Input: part model. Units: mm. Frame: model coordinates. A direction names the side the tool comes from. Give positions to 0.01 mm unless a question says otherwise; leave off trailing zeros. Loops run counter-clockwise (first coordinate to the right, second up) from the corner with the lowest first, then second, coordinate; pieces in that order, holes last. Notation, with made-up numbers: (32.25, 75) - (87.25, 75) arc R18 ccw to (87.25, 107) - close; hole circle Ø4 at (-21, 79). An arc over 180 degrees is marked (long way). Answer as a JSON object with one key per item and string values. Group by question number.
(1) Section query D-D (z = 6). Return loops of the section in (x, y) (3 decimals).
(2) Access query for faces 4 (the cylindrical face through (-7.074, 7.09, 7.535)), 5 (the flat face through (-7.375, 0, 7)), 6 (the flat face through (6.375, 0, 6)), 7 (the cylindrical face through (7.09, 7.074, 7.535)). Directions: +Z, -Z, +X, -X, +Y, -Y. A direction counts if a zero-diameter tool reaches every point of the face in a straight line with its end or side. Return the directions, or none.
(3) Mould query, pull axis Y, two halves, no side actions, for faces 1 (the flat face through (0, 0, 2)), 2 (the cylindrical face through (14.1, -14.14, 2.54)), 3 (the flat face through (0, 10, 5)). Classes: +Y half, -Y half, draft (parallel to the pull), parting line (faces both ways), or undercut.
(4) Section query B-B (y = 5). Return loops of the section in (x, z) (3 decimals).
(5) Section query A-A (z = 3). Return loops of the section in (x, y) (3 decimals).
(6) Material intervals for L1, parallel to X at y = 0.75, z = 4.5 (3 decimals); L2, parallel to Y at x = 0, z = 7.25 (3 decimals), sorted ascending.
(7) Section query C-C (x = 6.75). Return loops of the section in (y, z), plus the area to 3 significant figures.
(8) Pin query (flat end, axial travel): P1, Ø4, axis at y = -0.5, z = 7.5, coming from the -X side (3 decimals); P2, Ø1.5, axis at y = -2.5, z = 7, coming from the +X side (3 decimals); P3, Ø2.5, axis at x = -2.5, z = 7.5, coming from the +Y side (3 decimals). Return the tip coordinate at first contact, or that it passes through.
Autodesk Fusion 360 part; units mm, degrees
sketch "Sketch1" plane through (0, 0, 0) normal (0, 0, 1) x (1, 0, 0)
  line L0 (15, -15) -> (-15, -15)
  line L1 (-15, -15) -> (-15, 15)
  line L2 (-15, 15) -> (15, 15)
  line L3 (15, 15) -> (15, -15)
  line L4 (15, -15) -> (-15, 15) construction
  line L5 (-15, -15) -> (15, 15) construction
  dimension "d1" = 30
  dimension "d2" = 30
extrude "Extrude1" add sketch "Sketch1" along normal blind 5 makes body 1
sketch "Sketch2" plane through (0, 0, 5) normal (0, 0, 1) x (-1, 0, 0)
  line L0 (-15, -15) -> (15, -15)
  line L1 (15, -15) -> (15, 15)
  line L2 (15, 15) -> (-15, 15)
  line L3 (-15, 15) -> (-15, -15)
  line L4 (6.375, -6.375) -> (-6.375, -6.375)
  line L5 (-6.375, -6.375) -> (-6.375, 6.375)
  line L6 (-6.375, 6.375) -> (6.375, 6.375)
  line L7 (6.375, 6.375) -> (6.375, -6.375)
  line L8 (6.375, -6.375) -> (-6.375, 6.375) construction
  line L9 (-6.375, -6.375) -> (6.375, 6.375) construction
  line L10 (7.375, 7.375) -> (7.375, -7.375)
  line L11 (7.375, -7.375) -> (-7.375, -7.375)
  line L12 (-7.375, -7.375) -> (-7.375, 7.375)
  line L13 (-7.375, 7.375) -> (7.375, 7.375)
  dimension "d5" = 12.75
  dimension "d6" = 12.75
  dimension "d7" = -1
extrude "Extrude2" add sketch "Sketch2" along normal blind 5 contours L10 L11 L12 L13 bodies 1
extrude "Extrude3" cut 1 faces at (-2.125, -2.125, 5) along direction (0, 0, -1) up to surface (3 mm away) on bodies 1 bodies 1
fillet "Fillet1" radius 3 1 edges at (-15, 15, 2.5) on bodies 1
fillet "Fillet2" radius 3 3 edges at (-15, -15, 2.5) (15, -15, 2.5) (15, 15, 2.5) on bodies 1
fillet "Fillet3" radius 1 4 edges at (7.375, 7.375, 7.5) (-7.375, 7.375, 7.5) (7.375, -7.375, 7.5) (-7.375, -7.375, 7.5) on bodies 1
copy_body "Body->Comp1" bodies 1 removing the originals makes body 2 in component "Cuvette_Holder"
component "Cuvette_Holder" placed x (1, 0, 0) y (0, 1, 0) z (0, 0, 1) at (0, 0, 0)
Recorded:
{
 "1": {"outline": "(-7.375, -6.375) arc R1 ccw to (-6.375, -7.375) - (6.375, -7.375) arc R1 ccw to (7.375, -6.375) - (7.375, 6.375) arc R1 ccw to (6.375, 7.375) - (-6.375, 7.375) arc R1 ccw to (-7.375, 6.375) - close; hole (-6.375, -6.375) - (6.375, -6.375) - (6.375, 6.375) - (-6.375, 6.375) - close"},
 "2": {"face 4": "+Z, -X, +Y", "face 5": "+Z, -X, +Y, -Y", "face 6": "+Z", "face 7": "+Z, +X, +Y"},
 "3": {"face 1": "undercut", "face 2": "-Y half", "face 3": "draft"},
 "4": {"outline": "(-15, 0) - (15, 0) - (15, 5) - (7.375, 5) - (7.375, 10) - (6.375, 10) - (6.375, 2) - (-6.375, 2) - (-6.375, 10) - (-7.375, 10) - (-7.375, 5) - (-15, 5) - close"},
 "5": {"outline": "(-15, -12) arc R3 ccw to (-12, -15) - (12, -15) arc R3 ccw to (15, -12) - (15, 12) arc R3 ccw to (12, 15) - (-12, 15) arc R3 ccw to (-15, 12) - close; hole (-6.375, -6.375) - (6.375, -6.375) - (6.375, 6.375) - (-6.375, 6.375) - close"},
 "6": {"L1": "x = -15 to -6.375, 6.375 to 15", "L2": "y = -7.375 to -6.375, 6.375 to 7.375"},
 "7": {"outline": "(-15, 0) - (15, 0) - (15, 5) - (7.3, 5) - (7.3, 10) - (-7.3, 10) - (-7.3, 5) - (-15, 5) - close", "area": "223 mm^2"},
 "8": {"P1": "stops at x = -7.375", "P2": "stops at x = 7.375", "P3": "stops at y = 7.375"}
}
